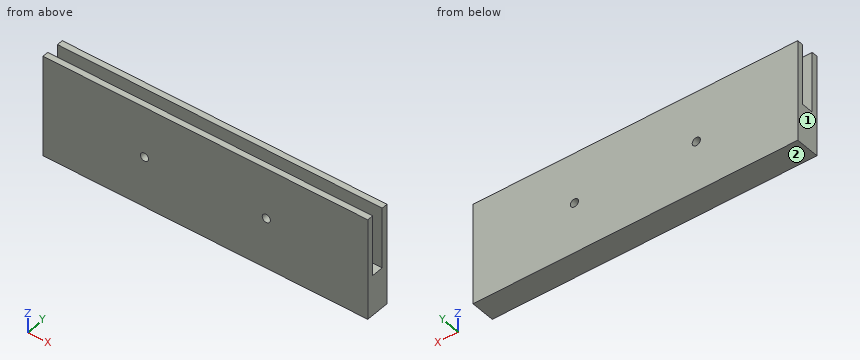
```python
from build123d import *

# Parameters (mm, degrees)
CROQUIS1_W                 = 80
CROQUIS1_H                 = 6
SALIENTE_EXTRUIR4_DEPTH    = 10
CROQUIS5_W                 = 80
CROQUIS5_H                 = 6
SALIENTE_EXTRUIR6_DEPTH    = 10
CROQUIS7_W                 = 80
CROQUIS7_H                 = 1.5
SALIENTE_EXTRUIR7_DEPTH    = 10
CROQUIS9_W                 = 5
CROQUIS9_H                 = 3
CORTAR_EXTRUIR3_DEPTH      = 80
CROQUIS12_W                = 80
CROQUIS12_H                = 6
CORTAR_EXTRUIR4_DEPTH      = 10
CROQUIS13_W                = 80
CROQUIS13_H                = 6
SALIENTE_EXTRUIR8_DEPTH    = 5
CROQUIS14_R                = 1
CORTAR_EXTRUIR5_DEPTH      = 25
CROQUIS15_R                = 1
SALIENTE_EXTRUIR9_DEPTH    = 1
SALIENTE_EXTRUIR10_START   = -1
CROQUIS16_R                = 1
SALIENTE_EXTRUIR10_DEPTH   = 1
CORTAR_EXTRUIR6_DEPTH      = 86.650452421
CORTAR_EXTRUIR6_DEPTH_BACK = 25
CROQUIS17_R                = 1


with BuildPart() as part:
    # Croquis1 → Saliente-Extruir4 (new body)
    with BuildSketch(Plane.XY):
        with Locations((40, 3)):
            Rectangle(CROQUIS1_W, CROQUIS1_H)
    extrude(amount=SALIENTE_EXTRUIR4_DEPTH)

    # Croquis5 → Saliente-Extruir6 (add)
    with BuildSketch(Plane.XY.offset(10)):
        with Locations((40, 3)):
            Rectangle(CROQUIS5_W, CROQUIS5_H)
    extrude(amount=SALIENTE_EXTRUIR6_DEPTH)

    # Croquis7 → Saliente-Extruir7 (add)
    with BuildSketch(Plane.XY.offset(20)):
        with Locations((40, 5.25)):
            Rectangle(CROQUIS7_W, CROQUIS7_H)
        with Locations((40, 0.75)):
            Rectangle(CROQUIS7_W, CROQUIS7_H)
    extrude(amount=SALIENTE_EXTRUIR7_DEPTH)

    # Croquis9 → Cortar-Extruir3 (cut)
    with BuildSketch(Plane.ZY):
        with Locations((17.5, 3)):
            Rectangle(CROQUIS9_W, CROQUIS9_H)
    extrude(amount=-CORTAR_EXTRUIR3_DEPTH, mode=Mode.SUBTRACT)

    # Croquis12 → Cortar-Extruir4 (cut)
    with BuildSketch(Plane(origin=(0, 0, 0), x_dir=(-1, 0, 0), z_dir=(0, 0, -1))):
        with Locations((-40, 3)):
            Rectangle(CROQUIS12_W, CROQUIS12_H)
    extrude(amount=-CORTAR_EXTRUIR4_DEPTH, mode=Mode.SUBTRACT)

    # Croquis13 → Saliente-Extruir8 (add)
    with BuildSketch(Plane(origin=(0, 0, 10), x_dir=(-1, 0, 0), z_dir=(0, 0, -1))):
        with Locations((-40, 3)):
            Rectangle(CROQUIS13_W, CROQUIS13_H)
    extrude(amount=SALIENTE_EXTRUIR8_DEPTH)

    # Croquis14 → Cortar-Extruir5 (cut)
    with BuildSketch(Plane(origin=(0, 6, 0), x_dir=(1, 0, 0), z_dir=(0, 1, 0))):
        with Locations(Location((20, -17.5, 0), (0, 0, 270))):
            Circle(CROQUIS14_R)
        with Locations(Location((60, -17.5, 0), (0, 0, 270))):
            Circle(CROQUIS14_R)
    extrude(amount=-CORTAR_EXTRUIR5_DEPTH, mode=Mode.SUBTRACT)

    # Croquis15 → Saliente-Extruir9 (add)
    with BuildSketch(Plane(origin=(0, 6, 0), x_dir=(1, 0, 0), z_dir=(0, 1, 0))):
        with Locations(Location((20, -17.5, 0), (0, 0, 270))):
            Circle(CROQUIS15_R)
        with Locations(Location((60, -17.5, 0), (0, 0, 270))):
            Circle(CROQUIS15_R)
    extrude(amount=-SALIENTE_EXTRUIR9_DEPTH)

    # Croquis16 → Saliente-Extruir10 (add)
    with BuildSketch(Plane.XZ.offset(SALIENTE_EXTRUIR10_START)):
        with Locations(Location((20, 17.5, 0), (0, 0, 270))):
            Circle(CROQUIS16_R)
        with Locations(Location((60, 17.5, 0), (0, 0, 270))):
            Circle(CROQUIS16_R)
    extrude(amount=SALIENTE_EXTRUIR10_DEPTH)

    # Croquis17 → Cortar-Extruir6 (cut, two sides: drawn at the far end of the back side and taken through both)
    with BuildSketch(Plane(origin=(0, 6, 0), x_dir=(1, 0, 0), z_dir=(0, 1, 0)).offset(-CORTAR_EXTRUIR6_DEPTH_BACK)):
        with Locations(Location((25, -17.5, 0), (0, 0, 90))):
            Circle(CROQUIS17_R)
        with Locations(Location((55, -17.5, 0), (0, 0, 90))):
            Circle(CROQUIS17_R)
    extrude(amount=CORTAR_EXTRUIR6_DEPTH + CORTAR_EXTRUIR6_DEPTH_BACK, mode=Mode.SUBTRACT)


solid = part.part
```
Verification items for the finished model (mm, model axes). Face numbers are marked on the shaded views. Give positions to 0.01 mm unless a question says otherwise; leave off trailing zeros. Order: outer loops, then holes, each group sorted by start corner. A loop starts at its lowest first (then second) coordinate and runs counter-clockwise, first axis right, second up. Notation, with made-up numbers: (46.5, 29.5) - (88.5, 29.5) arc R17 cw to (88.5, 62.5) - close; hole circle Ø9 at (-16, -0.75). An arc over 180 degrees is marked (long way). Answer as CSV lines item,"result". Start each with the question number.
Item 1: Mould release check, pull along Z, two halves, no side actions. Record for the marked faces 1 and 2: released by +Z, released by -Z, zero draft, split by the parting line, or undercut.
Item 2: Section check A-A, the plane x = 25. Record the boundary of the cut face in (y, z), plus the area to 3 significant figures.
Item 3: Section check B-B, the plane x = 60. Record the boundary of the cut face in (y, z).
Item 4: Section check D-D, the plane y = 3.2. Record the boundary of the cut face in (x, z), plus the area to 3 significant figures.
Item 5: Material ranges on L1, parallel to X at y = 5.1, z = 17.5; L2, parallel to X at y = 4.6, z = 17.5; L3, parallel to Y at x = 15, z = 18.5, recorded low to high.
Item 6: Section check C-C, the plane z = 17.5. State how many separate pieces and enclosed holes the cut face has, plus the area to 3 significant figures.
Filled in:
1,face 1,"zero draft"
1,face 2,"released by -Z"
2,outline,"(0, 5) - (6, 5) - (6, 16.5) - (4.5, 16.5) - (4.5, 15) - (1.5, 15) - (1.5, 16.5) - (0, 16.5) - close; (0, 18.5) - (1.5, 18.5) - (1.5, 30) - (0, 30) - close; (4.5, 18.5) - (6, 18.5) - (6, 30) - (4.5, 30) - close"
2,area,"99.0 mm^2"
3,outline,"(0, 5) - (6, 5) - (6, 30) - (4.5, 30) - (4.5, 18.5) - (5, 18.5) - (5, 16.5) - (4.5, 16.5) - (4.5, 15) - (1.5, 15) - (1.5, 16.5) - (1, 16.5) - (1, 18.5) - (1.5, 18.5) - (1.5, 30) - (0, 30) - close"
4,outline,"(0, 5) - (80, 5) - (80, 15) - (0, 15) - close"
4,area,"800 mm^2"
5,L1,"0 to 24, 26 to 54, 56 to 80"
5,L2,"0 to 19, 21 to 24, 26 to 54, 56 to 59, 61 to 80"
5,L3,"0 to 1.5, 4.5 to 6"
6,separate pieces,"6"
6,enclosed holes,"0"
6,area,"224 mm^2"
